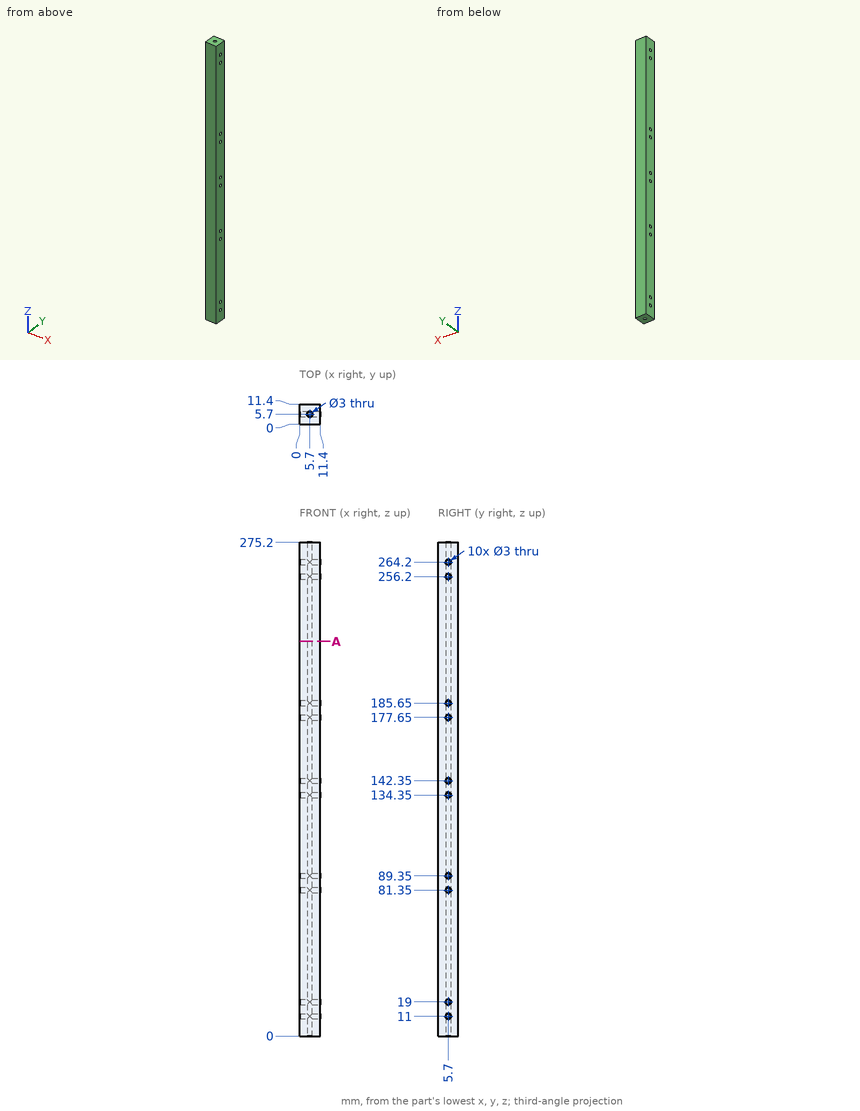
Can you work these out from the drawing? Everything is in mm from the part's minimum corner. Coordinates: 2 decimals unless noted, no trailing zeros. Order: outer loops, then holes, each group sorted by start corner. A loop starts at its lowest first (then second) coordinate and runs counter-clockwise, first axis right, second up. Notation, with made-up numbers: (36, -30.5) -> (49, -30.5) arc R32 ccw to (49, 6.5) -> close; hole circle Ø3 at (-14.5, 64.5). An arc over 180 degrees is marked (long way). Return JSON: item names as keys, results as strings.
1) If I drill on probe 1 along Y at (x, z) = (5.75, 97.5); probe 2 along X at (y, z) = (4.75, 227), over which ranges is the centre line in solid material (lowest first)?
Conclusion:
{"probe 1": "y = 0 to 4.2, 7.2 to 11.4", "probe 2": "x = 0 to 4.54, 6.86 to 11.4"}
2) If we section it at A-A on z = 220: List the corners of the cut face in (x, y) for me, plus the area to 3 significant figures.
Conclusion:
{"outline": "(0, 0) -> (11.4, 0) -> (11.4, 11.4) -> (0, 11.4) -> close; hole circle Ø3 at (5.7, 5.7)", "area": "123 mm²"}
3) I'm going to push a flat-ended pin straight in: P1, Ø2.5, axis at y = 5.7, z = 81.35, coming from the +X side. Where does the tip first touch, or does it pass through?
Conclusion:
{"P1": "passes through"}
